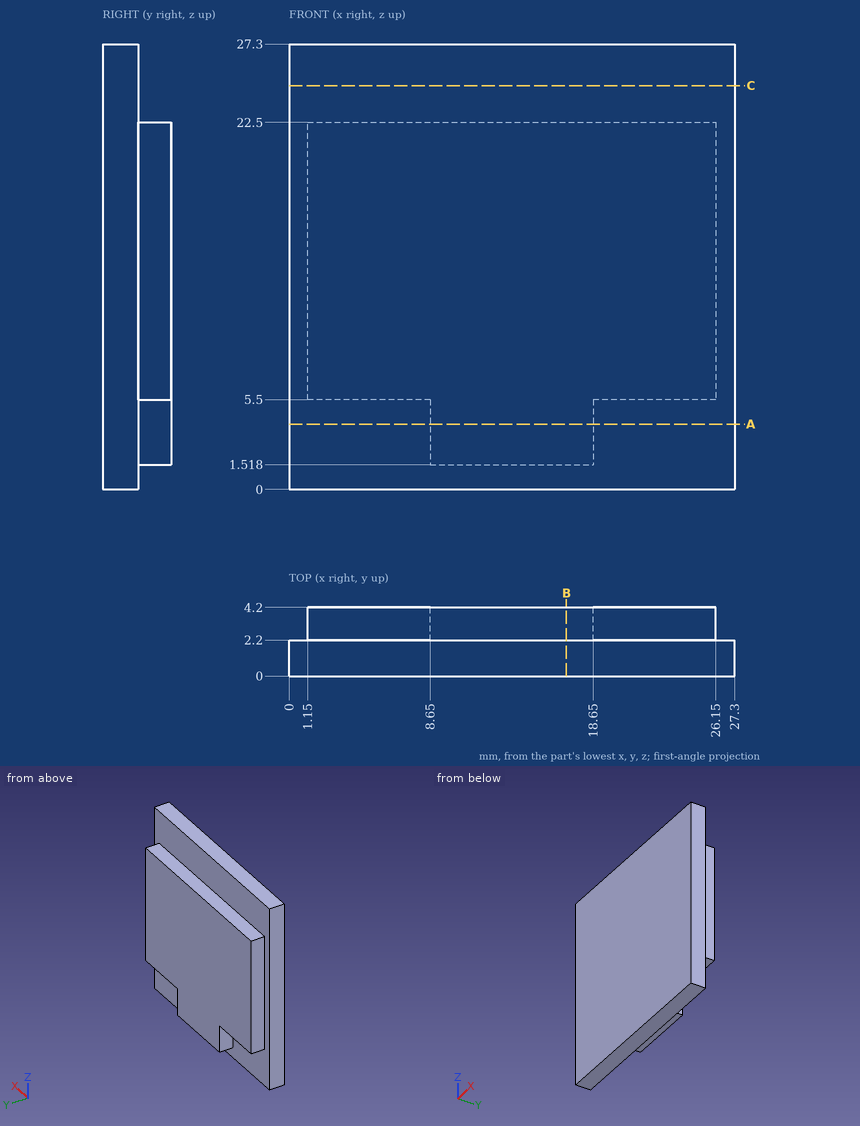
Geometry: see drawing. Coordinates: mm, zero at the bounding-box minimum. Give positions to 0.01 mm unless a question says otherwise; leave off trailing zeros. Order: outer loops, then holes, each group sorted by start corner. A loop starts at its lowest first (then second) coordinate and runs counter-clockwise, first axis right, second up. Notation, with made-up numbers: (-31.5, -7.75) - (15.5, -7.75) arc R32 ccw to (15.5, 23.25) - close; hole circle Ø4 at (-3.5, 75). An arc over 180 degrees is marked (long way). Write each question's results on one line, items separated by ' | '.
Item 1: Contact query for flat-ended pins moving along their axis: pin 1 Ø1 at (y, z) = (3, 2.5) entering from +X; pin 2 Ø1.6 at (y, z) = (3.5, 11.5) entering from +X; pin 3 Ø1 at (x, y) = (16, 3.5) entering from -Z. Output: stop coordinate, or through.
A:
pin 1: stops at x = 18.65 | pin 2: stops at x = 26.15 | pin 3: stops at z = 1.52
Item 2: Material intervals for line 1 along X through (y, z) = (2.75, 8.5); line 2 along Z through (x, y) = (11.75, 3.35); line 3 along Z through (x, y) = (21, 3.9), sorted ascending.
A:
line 1: x = 1.15 to 26.15 | line 2: z = 1.52 to 22.5 | line 3: z = 5.5 to 22.5
Item 3: Section A-A (z = 4). Return loops of the section in (x, y).
A:
outline: (0, 0) - (27.3, 0) - (27.3, 2.2) - (18.65, 2.2) - (18.65, 4.2) - (8.65, 4.2) - (8.65, 2.2) - (0, 2.2) - close
Item 4: Section B-B (x = 17). Return loops of the section in (y, z).
A:
outline: (0, 0) - (2.2, 0) - (2.2, 1.52) - (4.2, 1.52) - (4.2, 22.5) - (2.2, 22.5) - (2.2, 27.3) - (0, 27.3) - close
Item 5: Section C-C (z = 24.75). Return loops of the section in (x, y).
A:
outline: (0, 0) - (27.3, 0) - (27.3, 2.2) - (0, 2.2) - close
